CAD build for the part. Positions are in the model's coordinates, mm. Face numbers are marked on the shaded views. A direction names the side the tool comes from. Give positions to 0.01 mm unless a question says otherwise; leave off trailing zeros. Write each loop counter-clockwise with the first axis right and the second up, starting at its lowest first coordinate (ties: lowest second). Pieces come first, ordered by that corner, then holes. Notation, with made-up numbers: M 33.25,63.5 L 63.25,63.5 A10 cw 63.25,74.5 Z; hole C 24.5,86.25 d10. An arc over 180 degrees is marked long. One line per question, with ' | ' between items. Start each with the question number.
1. Pull direction Z, two halves, no side cores. Call the marked faces 1, 2, 3 and 4: released by +Z, released by -Z, zero draft, split by the parting line, or undercut.
2. Wall check: L1, parallel to X at y = -369, z = 133.5; L2, parallel to Z at x = -68, y = -329; L3, parallel to Z at x = -127, y = -445. Give the ranges that are in metal, low to high.
3. Cut at B-B, the plane y = -53. Write the cut outline in (x, z), then the cut area to 3 significant figures.
4. Cut at D-D, the plane x = -128. Write the cut outline in (y, z), then the cut area to 3 significant figures.
5. Which spindle directions (+Z, -Z, +X, -X, +Y, -Y) get a long thin tool onto all of the face, cutting with end or side? Do the marked faces 5 and 6. Say none if no direction does.
6. Cut at A-A, the plane x = -211. Write the cut outline in (y, z), then the cut area to 3 significant figures.
7. Cut at C-C, the plane z = 70. Write the cut outline in (x, y).
8. Flat gauge pin, fed straight in: pin 1 (3 mm diameter, centred on x = -69, y = -168.5, fed in from +Z). Where does the tip first touch, or does it go through?
```python
from build123d import *

# Parameters (mm, degrees)
F1_DEPTH = 19.05
F2_DEPTH = 609.6
F3_E0_W  = 1524
F3_E0_H  = 609.6
F4_DEPTH = 19.05
F5_DEPTH = 25.4
F6_E4_W  = 207.3184425354
F6_E4_H  = 609.6
F7_DEPTH = 19.05


with BuildPart() as f1:
    # F0 (on Front) → F1 (new body)
    with BuildSketch(Plane.XZ):
        Polygon((-24.7226779938, -763.8654754907), (-24.7226779938, -474.9317169189), (-227.9226779938, -763.8654754907), align=None)
    extrude(amount=F1_DEPTH)

    # F0 (on Front) → F2 (join)
    with BuildSketch(Plane.XZ):
        Polygon((-24.7226779938, -763.8654754907), (-24.7226779938, -474.9317169189), (-227.9226779938, -763.8654754907), align=None)
    extrude(amount=F2_DEPTH)

    # F3_E0 (on explicit) → F4 (join)
    with BuildSketch(Plane(origin=(-24.7226779938, 0, 760.1345245093), x_dir=(0, 0, -1), z_dir=(-1, 0, 0))):
        with Locations((762, 304.8)):
            Rectangle(F3_E0_W, F3_E0_H)
    extrude(amount=F4_DEPTH)

    # F0 (on Front) → F5 (join)
    with BuildSketch(Plane.XZ):
        Polygon((-24.7226779938, -763.8654754907), (-24.7226779938, -474.9317169189), (-227.9226779938, -763.8654754907), align=None)
    extrude(amount=F5_DEPTH)

    # F6_E4 (on explicit) → F7 (join)
    with BuildSketch(Plane(origin=(-24.7226779938, 0, -348.2956886292), x_dir=(-1, 0, 0), z_dir=(0, 0, 1))):
        with Locations((103.6592212677, 304.8)):
            Rectangle(F6_E4_W, F6_E4_H)
    extrude(amount=F7_DEPTH)


solid = f1.part
```
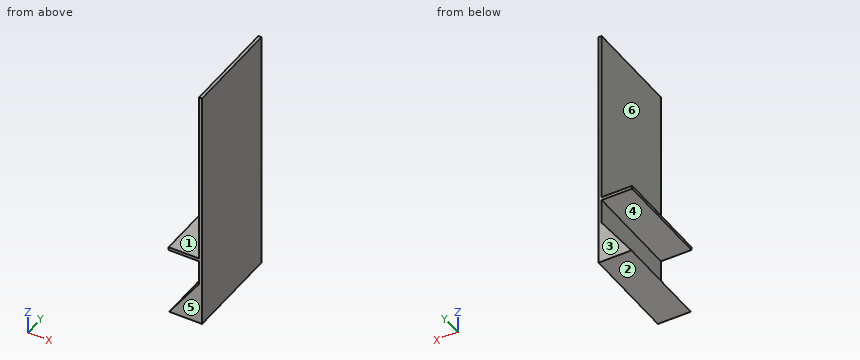
Here are the results:
1) face 1: released by +Z | face 2: released by -Z | face 3: zero draft | face 4: undercut
2) L1: -43.77 to -24.72 | L2: -763.87 to -536.47, -348.3 to -329.25 | L3: -763.87 to -620.36, -348.3 to -329.25
3) outline: M -232.04,-348.3 L -43.77,-348.3 L -43.77,-502.02 L -227.92,-763.87 L -24.72,-763.87 L -24.72,760.13 L -43.77,760.13 L -43.77,-329.25 L -232.04,-329.25 Z | area: 56,700 mm^2
4) outline: M -609.6,-763.87 L 0,-763.87 L 0,-621.78 L -609.6,-621.78 Z; M -609.6,-348.3 L 0,-348.3 L 0,-329.25 L -609.6,-329.25 Z | area: 98,200 mm^2
5) face 5: +Z, -Z, +X, -X, -Y | face 6: +Z, -X, +Y, -Y
6) outline: M -609.6,-763.87 L 0,-763.87 L 0,-739.8 L -609.6,-739.8 Z; M -609.6,-348.3 L 0,-348.3 L 0,-329.25 L -609.6,-329.25 Z | area: 26,300 mm^2
7) outline: M -43.77,-609.6 L -24.72,-609.6 L -24.72,0 L -43.77,0 Z
8) pin 1: z = -329.25
